Could you check a few things on this model? Use its own coordinates, in mm. Face numbers are marked on the shaded views. A direction names the side the tool comes from. Coordinates: 2 decimals unless noted, no trailing zeros. Order: outer loops, then holes, each group sorted by start corner. A loop starts at its lowest first (then second) coordinate and runs counter-clockwise, first axis right, second up. Notation, with made-up numbers: (83, 7) - (122, 7) arc R34 cw to (122, 44) - close; hole circle Ø7 at (8, 4.5). An arc over 180 degrees is marked (long way). Answer as a JSON object with one key per item and string values. Group by question number.
(1) Please list where these lines run through material, in increasing order: probe 1 along Z at (x, y) = (-32, 12); probe 2 along X at (y, z) = (5, -6.5); probe 3 along Z at (x, y) = (-67, 7).
(2) Imagine slicing it at C-C, the plane z = 6.5. Write out the boundary of the cut face in (x, y).
(3) Imagine slicing it at D-D, the plane y = 10.5. Give the number of separate pieces and of enclosed holes in the cut face, and give its area (3 significant figures).
(4) Will these pins go through, and if not, where does the flat tip stop? P1, Ø5, axis at y = 13, z = 15, coming from the +X side; P2, Ø22, axis at x = -18.5, z = 1, coming from the +Y side; P3, Ø8.5, axis at x = 75, z = 4, coming from the +Y side.
(5) Imagine slicing it at A-A, the plane z = -25.1. Write out the boundary of the cut face in (x, y), and give its area (3 significant figures).
(6) Which directions (+Z, -Z, +X, -X, +Y, -Y) give clear straight access to the entire face, cutting with the end or side of a thin tool? Please do the marked faces 1 and 2.
(7) We'd pull the mould along X, two halves only. Please class the marked faces 3, 4 and 5: pulls with the +X half, pulls with the -X half, needs draft (parallel to the pull), parting line crosses it, or undercut.
(8) Imagine slicing it at B-B, the plane x = -22. Write out the boundary of the cut face in (y, z), and give its area (3 significant figures).
from build123d import *

# Parameters (mm, degrees)
EXTRUDE_1_DEPTH     = 15
CUT_EXTRUDE_1_DEPTH = 11
EXTRUDE_2_DEPTH     = 11
SKETCH_4_R          = 2.1
CUT_EXTRUDE_2_DEPTH = 91.691785736
FILLET_1_R          = 3
CUT_EXTRUDE_3_REACH = 167.605
SKETCH_5_W          = 40
SKETCH_5_H          = 40


with BuildPart() as part:
    # Эскиз1 → Бобышка-Вытянуть1 (new body)
    with BuildSketch(Plane(origin=(0, 0, 0), x_dir=(1, 0, 0), z_dir=(0, 1, 0))):
        with BuildLine():
            Line((-77, -40), (77, -40))
            ThreePointArc((77, -40), (79.121320344, -39.121320344), (80, -37))
            Line((80, -37), (80, 37))
            ThreePointArc((80, 37), (79.121320344, 39.121320344), (77, 40))
            Line((77, 40), (-77, 40))
            ThreePointArc((-77, 40), (-79.121320344, 39.121320344), (-80, 37))
            Line((-80, 37), (-80, -37))
            ThreePointArc((-80, -37), (-79.121320344, -39.121320344), (-77, -40))
        make_face()
    extrude(amount=EXTRUDE_1_DEPTH)

    # Эскиз2 → Вырез-Вытянуть1 (cut)
    with BuildSketch(Plane(origin=(0, 15, 0), x_dir=(1, 0, 0), z_dir=(0, 1, 0))):
        with BuildLine():
            Line((-75.75, -36.7), (75.75, -36.7))
            ThreePointArc((75.75, -36.7), (76.457106781, -36.407106781), (76.75, -35.7))
            Line((76.75, -35.7), (76.75, 35.7))
            ThreePointArc((76.75, 35.7), (76.457106781, 36.407106781), (75.75, 36.7))
            Line((75.75, 36.7), (-75.75, 36.7))
            ThreePointArc((-75.75, 36.7), (-76.457106781, 36.407106781), (-76.75, 35.7))
            Line((-76.75, 35.7), (-76.75, -35.7))
            ThreePointArc((-76.75, -35.7), (-76.457106781, -36.407106781), (-75.75, -36.7))
        make_face()
    extrude(amount=-CUT_EXTRUDE_1_DEPTH, mode=Mode.SUBTRACT)

    # Эскиз3 → Бобышка-Вытянуть2 (add)
    with BuildSketch(Plane(origin=(0, 4, 0), x_dir=(1, 0, 0), z_dir=(0, 1, 0))):
        with BuildLine():
            Line((-76.75, -36.7), (-68.2, -36.7))
            Line((-68.2, -36.7), (-68.2, -22.15))
            ThreePointArc((-68.2, -22.15), (-69.078679656, -20.028679656), (-71.2, -19.15))
            Line((-71.2, -19.15), (-76.75, -19.15))
            Line((-76.75, -19.15), (-76.75, -36.7))
        make_face()
        with BuildLine():
            Line((-68.2, 36.7), (-68.2, 22.15))
            ThreePointArc((-68.2, 22.15), (-69.078679656, 20.028679656), (-71.2, 19.15))
            Line((-71.2, 19.15), (-76.75, 19.15))
            Line((-76.75, 19.15), (-76.75, 36.7))
            Line((-76.75, 36.7), (-68.2, 36.7))
        make_face()
        with BuildLine():
            Line((76.75, 36.7), (68.2, 36.7))
            Line((68.2, 36.7), (68.2, 22.15))
            ThreePointArc((68.2, 22.15), (69.078679656, 20.028679656), (71.2, 19.15))
            Line((71.2, 19.15), (76.75, 19.15))
            Line((76.75, 19.15), (76.75, 36.7))
        make_face()
        with BuildLine():
            Line((68.2, -36.7), (68.2, -22.15))
            ThreePointArc((68.2, -22.15), (69.078679656, -20.028679656), (71.2, -19.15))
            Line((71.2, -19.15), (76.75, -19.15))
            Line((76.75, -19.15), (76.75, -36.7))
            Line((76.75, -36.7), (68.2, -36.7))
        make_face()
    extrude(amount=EXTRUDE_2_DEPTH)

    # Эскиз4 → Вырез-Вытянуть2 (cut, through all)
    with BuildSketch(Plane(origin=(0, 15, 0), x_dir=(1, 0, 0), z_dir=(0, 1, 0))):
        with Locations(Location((-74.15, -34, 0), (0, 0, 270))):
            Circle(SKETCH_4_R)
        with Locations(Location((-74.15, 34, 0), (0, 0, 90))):
            Circle(SKETCH_4_R)
        with Locations(Location((74.15, 34, 0), (0, 0, 270))):
            Circle(SKETCH_4_R)
        with Locations(Location((74.15, -34, 0), (0, 0, 90))):
            Circle(SKETCH_4_R)
        with Locations(Location((-74.15, -25.1, 0), (0, 0, 270))):
            Circle(SKETCH_4_R)
        with Locations(Location((-74.15, 25.1, 0), (0, 0, 90))):
            Circle(SKETCH_4_R)
        with Locations(Location((74.15, 25.1, 0), (0, 0, 270))):
            Circle(SKETCH_4_R)
        with Locations(Location((74.15, -25.1, 0), (0, 0, 90))):
            Circle(SKETCH_4_R)
    extrude(amount=-CUT_EXTRUDE_2_DEPTH, mode=Mode.SUBTRACT)

    # Скругление1
    fillet_1_edges = [part.edges().sort_by_distance(p)[0] for p in [
        (76.75, 9.5, 19.15),
        (68.2, 9.5, 36.7),
        (-68.2, 9.5, 36.7),
        (-76.75, 9.5, 19.15),
        (-76.75, 9.5, -19.15),
        (-68.2, 9.5, -36.7),
        (68.2, 9.5, -36.7),
        (76.75, 9.5, -19.15),
    ]]
    fillet(fillet_1_edges, radius=FILLET_1_R)

    # Вырез-Вытянуть3: up to this face of the body (flat: up to its plane)
    cut_extrude_3_end = Plane(part.part.faces().sort_by_distance((68.2, 9.5, -27.925))[0])
    # Эскиз5 → Вырез-Вытянуть3 (cut, up to the picked face)
    with BuildSketch(Plane(origin=(80, 0, 0), x_dir=(0, 0, -1), z_dir=(1, 0, 0)), mode=Mode.PRIVATE) as cut_extrude_3_sk1:
        with Locations((0, 27.5)):
            Rectangle(SKETCH_5_W, SKETCH_5_H)
    cut_extrude_3_tool1 = split(extrude(cut_extrude_3_sk1.sketch, amount=-CUT_EXTRUDE_3_REACH, mode=Mode.PRIVATE), bisect_by=cut_extrude_3_end, keep=Keep.BOTH, mode=Mode.PRIVATE)
    add(cut_extrude_3_tool1.solids().sort_by(Axis((80, 27.5, 0), (-1, 0, 0)))[0], mode=Mode.SUBTRACT)


solid = part.part
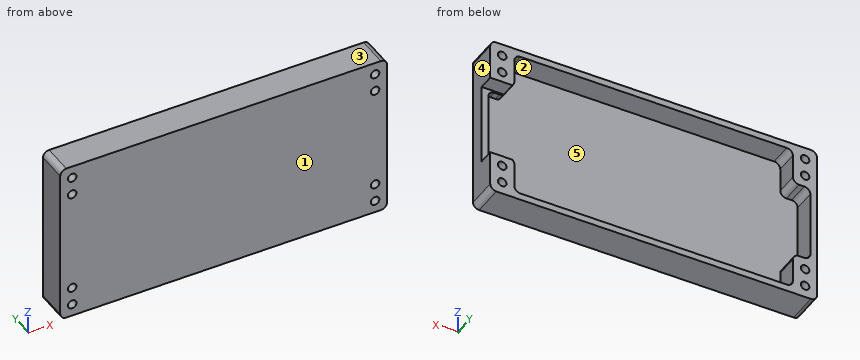
Result set:
{
 "1": {"probe 1": "z = -40 to -36.7, 36.7 to 40", "probe 2": "x = -80 to -76.75, 76.75 to 80", "probe 3": "z = -40 to -36.1, 36.1 to 40"},
 "2": {"outline": "(-80, 0) - (80, 0) - (80, 7.5) - (76.75, 7.5) - (76.75, 4) - (-76.75, 4) - (-76.75, 15) - (-80, 15) - close"},
 "3": {"separate pieces": "1", "enclosed holes": "8", "area": "1,880 mm^2"},
 "4": {"P1": "stops at x = -76.43", "P2": "stops at y = 4", "P3": "stops at y = 7.5"},
 "5": {"outline": "(-80, 0) - (-76.25, 0) - (-76.25, 15) - (-80, 15) - close; (-72.05, 0) - (72.05, 0) - (72.05, 15) - (68.2, 15) - (68.2, 4) - (-68.2, 4) - (-68.2, 15) - (-72.05, 15) - close; (76.25, 0) - (80, 0) - (80, 15) - (76.25, 15) - close", "area": "774 mm^2"},
 "6": {"face 1": "+Z, -Z, +X, -X, -Y", "face 2": "+Y"},
 "7": {"face 3": "needs draft", "face 4": "pulls with the +X half", "face 5": "undercut"},
 "8": {"outline": "(0, -40) - (15, -40) - (15, -36.7) - (4, -36.7) - (4, 36.7) - (15, 36.7) - (15, 40) - (0, 40) - close", "area": "393 mm^2"}
}
